Part model, mm, in its own coordinate system. A direction names the side the tool comes from. Coordinates: 2 decimals unless noted, no trailing zeros. Write each loop counter-clockwise with the first axis right and the second up, starting at its lowest first coordinate (ties: lowest second). Pieces come first, ordered by that corner, then holes. Notation, with made-up numbers: (-12, 58) - (17, 58) arc R32 ccw to (17, 85) - close; hole circle Ø11 at (5, 49.5). An arc over 180 degrees is marked (long way). Use a Markdown table: item, result.
```python
from build123d import *

# Parameters (mm, degrees)
SKETCH_1_W      = 4
SKETCH_1_H      = 50
EXTRUDE_1_DEPTH = 4


with BuildPart() as part:
    # Эскиз1 → Бобышка-Вытянуть1 (new body)
    with BuildSketch(Plane.XY):
        Polygon((-35.380363478, 50.607363696), (-65.380363478, 50.607363696), (-69.380363478, 50.607363696), (-69.380363478, -53.392636304), (-65.380363478, -53.392636304), (-35.380363478, -53.392636304), (-35.380363478, -49.392636304), (34.619636522, -49.392636304), (34.619636522, -53.392636304), (64.619636522, -53.392636304), (68.619636522, -53.392636304), (68.619636522, -24.392636304), (64.619636522, -24.392636304), (64.619636522, 25.607363696), (68.619636522, 25.607363696), (68.619636522, 50.607363696), (64.619636522, 50.607363696), (34.619636522, 50.607363696), (34.619636522, 54.607363696), (-35.380363478, 54.607363696), align=None)
        with Locations((36.619636522, 0.607363696)):
            Rectangle(SKETCH_1_W, SKETCH_1_H, mode=Mode.SUBTRACT)
    extrude(amount=EXTRUDE_1_DEPTH)


solid = part.part
```
Item 1: Drill centre lines: probe 1 along X at (y, z) = (1.5, 1.85); probe 2 along Y at (x, z) = (35, 1.25); probe 3 along Y at (x, z) = (54.5, 0.2). Where is each one in solid material? Low to high.
From the geometry:
| item | result |
|---|---|
| probe 1 | -69.38 to 34.62, 38.62 to 64.62 |
| probe 2 | -53.39 to -24.39, 25.61 to 50.61 |
| probe 3 | -53.39 to 50.61 |
Item 2: Band-saw the part on A-A, the plane z = 3.1. Give the cut face in (x, y).
From the geometry:
| item | result |
|---|---|
| outline | (-69.38, -53.39) - (-35.38, -53.39) - (-35.38, -49.39) - (34.62, -49.39) - (34.62, -53.39) - (68.62, -53.39) - (68.62, -24.39) - (64.62, -24.39) - (64.62, 25.61) - (68.62, 25.61) - (68.62, 50.61) - (34.62, 50.61) - (34.62, 54.61) - (-35.38, 54.61) - (-35.38, 50.61) - (-69.38, 50.61) - close; hole (34.62, -24.39) - (38.62, -24.39) - (38.62, 25.61) - (34.62, 25.61) - close |
Item 3: Two-plate mould, pull along X, no slides. Class faces 1 (the face through (-69.38, -1, 2)), 2 (the face through (34.62, 0, 2)), 3 (the face through (51, -53.393, 2)), 4 (the face through (34.62, -51, 2)): pulls with the +X half, pulls with the -X half, needs draft (parallel to the pull), parting line crosses it, or undercut.
From the geometry:
| item | result |
|---|---|
| face 1 | pulls with the -X half |
| face 2 | undercut |
| face 3 | needs draft |
| face 4 | undercut |
Item 4: Drop flat-ended pins along their axis: P1, Ø2, axis at x = 67, z = 2.5, coming from the +Y side; P2, Ø1.2, axis at y = 52.5, z = 3, coming from the -X side; P3, Ø1.2, axis at y = -8.5, z = 2.5, coming from the +X side. Give the stop position or say it passes through.
From the geometry:
| item | result |
|---|---|
| P1 | y = 50.61 |
| P2 | x = -35.38 |
| P3 | x = 64.62 |
Item 5: Which spindle directions (+Z, -Z, +X, -X, +Y, -Y) get a long thin tool onto all of the face, cutting with end or side? Do faces 5 (the face through (37, 25.607, 2)), 6 (the face through (-1, -49.393, 2)), 7 (the face through (67, -24.393, 2)). Say none if no direction does.
From the geometry:
| item | result |
|---|---|
| face 5 | +Z, -Z |
| face 6 | +Z, -Z, -Y |
| face 7 | +Z, -Z, +X |
Item 6: Band-saw the part on C-C, the plane x = -27.5. Give the cut face in (y, z), then the cut area to 3 significant figures.
From the geometry:
| item | result |
|---|---|
| outline | (-49.39, 0) - (54.61, 0) - (54.61, 4) - (-49.39, 4) - close |
| area | 416 mm^2 |
Item 7: Band-saw the part on B-B, the plane y = 23. Give the cut face in (x, z), then the cut area to 3 significant figures.
From the geometry:
| item | result |
|---|---|
| outline | (-69.38, 0) - (34.62, 0) - (34.62, 4) - (-69.38, 4) - close; (38.62, 0) - (64.62, 0) - (64.62, 4) - (38.62, 4) - close |
| area | 520 mm^2 |
